Build history of the part. All positions in model axes, mm. Face numbers are marked on the shaded views. A direction names the side the tool comes from. Give positions to 0.01 mm unless a question says otherwise; leave off trailing zeros. Loops run counter-clockwise (first coordinate to the right, second up) from the corner with the lowest first, then second, coordinate; pieces in that order, holes last.
1) Band-saw the part on A-A on y = 39.5. List the corners of the cut face in (x, z) (3 decimals), then the cut area to 3 significant figures.
2) Flat gauge pins, fed straight in: P1, Ø10, axis at x = 76, z = 55, coming from the -Y side; P2, Ø15.5, axis at x = 31.5, z = 36.5, coming from the +Y side; P3, Ø18.5, axis at y = -10, z = 6, coming from the +X side (3 decimals). Where does each tip first touch, or does it go through?
3) Wall check: line 1 (Y direction, x = -28.5, z = 16.5); line 2 (Z direction, x = -33, y = -52) (3 decimals); line 3 (Y direction, x = 29, z = 10). Give the ranges that are in metal, low to high.
4) Band-saw the part on B-B on x = 98. List the corners of the cut face in (y, z) (3 decimals).
5) 3-axis set-ups, long thin cutter, end or side, ignore diameter. For the marked faces 1, 2 and 3: which of +Z, -Z, +X, -X, +Y, -Y reach the whole face in a straight line?
```python
from build123d import *

# Parameters (mm, degrees)
F1_DEPTH = 63.5
F0_W     = 25.4
F0_H     = 19.05
F2_DEPTH = 25.4
F3_DEPTH = 7.9375


with BuildPart() as f1:
    # F0 (on Front) → F1 (new body, symmetric)
    with BuildSketch(Plane.XZ):
        Polygon((41.275, -9.525), (41.275, 9.525), (22.225, 9.525), (-41.275, 9.525), (-41.275, -9.525), align=None)
    extrude(amount=F1_DEPTH, both=True)

    # F0 (on Front) → F2 (join, symmetric)
    with BuildSketch(Plane.XZ):
        with Locations((73.025, 52.4002)):
            Rectangle(F0_W, F0_H)
        with BuildLine():
            Line((22.225, 9.525), (41.275, 9.525))
            Line((41.275, 9.525), (41.275, 27.0002))
            ThreePointArc((41.275, 27.0002), (45.9246798487, 38.2255201513), (57.15, 42.8752))
            Line((57.15, 42.8752), (60.325, 42.8752))
            Line((60.325, 42.8752), (60.325, 61.9252))
            Line((60.325, 61.9252), (57.15, 61.9252))
            add(Edge.make_bspline(
                [(56.5012045557, 61.9191732018), (56.7176813498, 61.9216130278), (56.9339488866, 61.9236220913), (57.15, 61.9252)],
                knots=[110.9630693968, 110.9630693968, 110.9630693968, 110.9630693968, 111.5045361635, 111.5045361635, 111.5045361635, 111.5045361635], degree=3))
            ThreePointArc((56.5012045557, 61.9191732018), (32.2259673619, 51.4654451869), (22.225, 27.0002))
            Line((22.225, 27.0002), (22.225, 9.525))
        make_face()
    extrude(amount=F2_DEPTH, both=True)

    # F0 (on Front) → F3 (join, symmetric)
    with BuildSketch(Plane.XZ):
        with BuildLine():
            Line((-41.275, 9.525), (22.225, 9.525))
            Line((22.225, 9.525), (22.225, 27.0002))
            ThreePointArc((22.225, 27.0002), (32.2259673619, 51.4654451869), (56.5012045557, 61.9191732018))
            add(Edge.make_bspline(
                [(-41.275, 9.525), (-41.0122764768, 42.8286605667), (12.1385012456, 61.4191783861), (56.5012045557, 61.9191732018)],
                knots=[0, 0, 0, 0, 110.9630693968, 110.9630693968, 110.9630693968, 110.9630693968], degree=3))
        make_face()
    extrude(amount=F3_DEPTH, both=True)

    # F0 (on Front) → F4 (revolve)
    with BuildSketch(Plane.XZ):
        Polygon((85.725, 61.9252), (85.725, 42.8752), (85.725, 38.1), (111.125, 38.1), (111.125, 66.675), (85.725, 66.675), align=None)
    revolve(axis=Axis((85.725, 0, 52.3875), (0, 0, 1)))


solid = f1.part
```
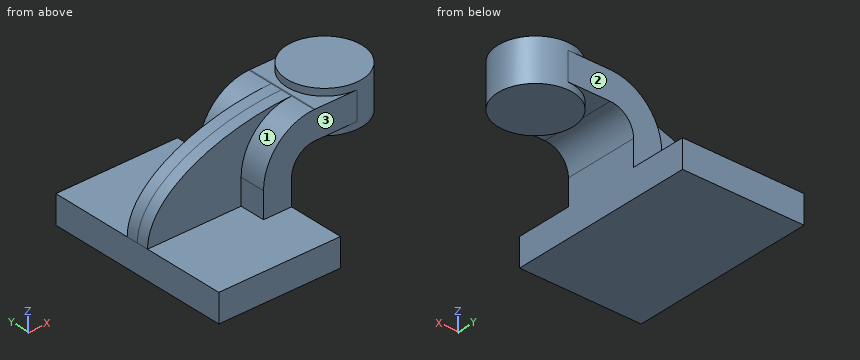
Findings below:
1. outline: (-41.275, -9.525) - (41.275, -9.525) - (41.275, 9.525) - (-41.275, 9.525) - close
1. area: 1,570 mm2
2. P1: stops at y = -25.4
2. P2: stops at y = 25.4
2. P3: stops at x = 41.275
3. line 1: y = -7.94 to 7.94
3. line 2: z = -9.525 to 9.525
3. line 3: y = -25.4 to 25.4
4. outline: (-22.237, 38.1) - (22.237, 38.1) - (22.237, 66.675) - (-22.237, 66.675) - close
5. face 1: +Z, -X, -Y
5. face 2: +Z, +X, -X, +Y
5. face 3: +Z, +X, -X, -Y
